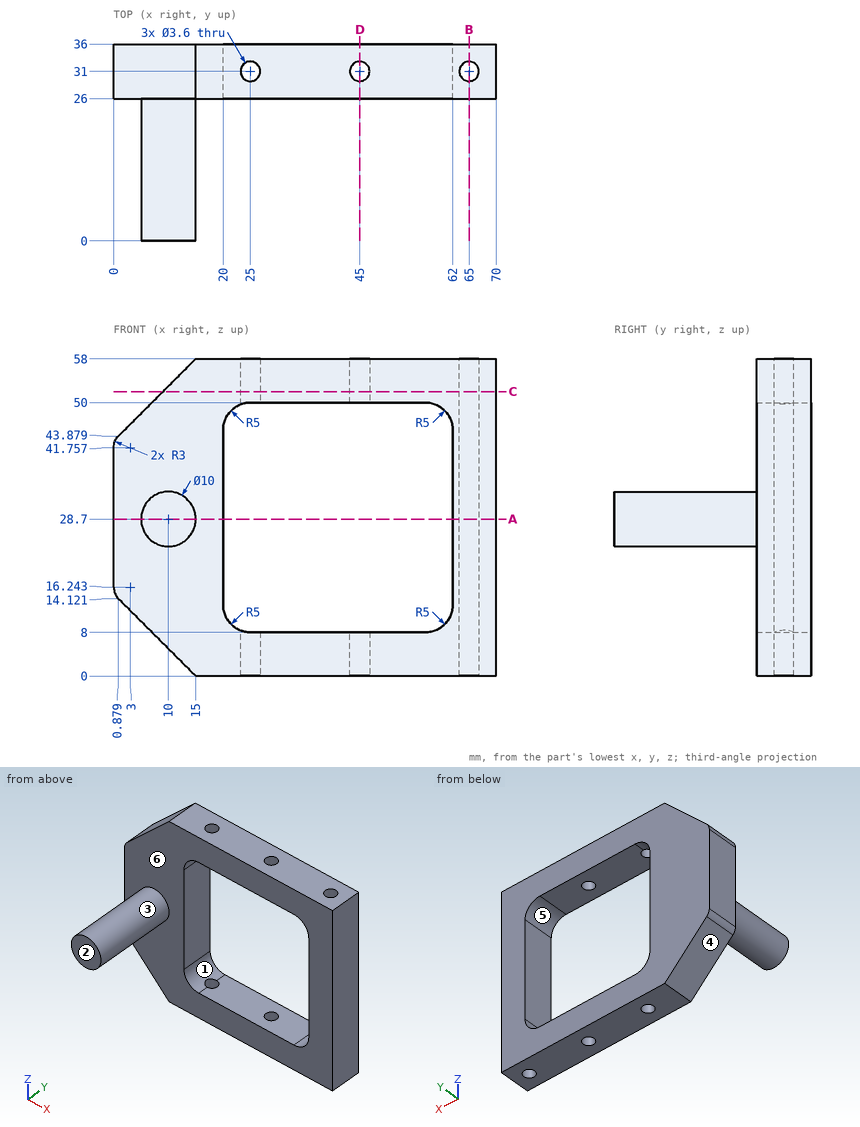
Verification items for this drawing (mm, ordinates from the low corner). A direction names the side the tool comes from. Round coordinates to 2 decimals unless told otherwise and drop trailing zeros. Loops run counter-clockwise (first coordinate to the right, second up) from the corner with the lowest first, then second, coordinate; pieces in that order, holes last. Notation, with made-up numbers: (22.25, 56.25) - (52.25, 56.25) arc R31 ccw to (52.25, 84.25) - close; hole circle Ø7 at (-28.5, 70). An arc over 180 degrees is marked (long way). Answer as CSV lines item,"result". Start each with the question number.
Item 1: Section check B-B (x = 65). Record the boundary of the cut face in (y, z), and give its area (3 significant figures).
Item 2: Section check A-A (z = 28.7). Record the boundary of the cut face in (x, y).
Item 3: Release check for a two-part mould opening along Z. For the marked faces 4, 5 and 6 record: +Z half, -Z half, draft (parallel to the pull), parting line (faces both ways), or undercut.
Item 4: Section check D-D (x = 45). Record the boundary of the cut face in (y, z).
Item 5: Scan lines: line 1 (Y direction, x = 45, z = 3.5); line 2 (X direction, y = 26.5, z = 34); line 3 (X direction, y = 31, z = 54). Record each from-to range of solid material in increasing order. Write a range as [from, to].
Item 6: Set-up check for the marked faces 1, 2 and 3: record each of +Z, -Z, +X, -X, +Y, -Y from which the full face is reachable in a straight line by a thin tool's end or side.
Item 7: Section check C-C (z = 52). Record the boundary of the cut face in (x, y).
Item 8: Depth check by flat-ended pin: P1, Ø3, axis at y = 23.5, z = 11, coming from the -X side; P2, Ø3, axis at x = 19.5, z = 39, coming from the -Y side; P3, Ø2, axis at y = 8, z = 29, coming from the -X side. Enter the tip coordinate at first touch or a pass-through.
Report:
1,outline,"(26, 0) - (29.2, 0) - (29.2, 58) - (26, 58) - close; (32.8, 0) - (36, 0) - (36, 58) - (32.8, 58) - close"
1,area,"371 mm2"
2,outline,"(0, 26) - (5, 26) - (5, 0) - (15, 0) - (15, 26) - (20, 26) - (20, 36) - (0, 36) - close; (62, 26) - (70, 26) - (70, 36) - (62, 36) - close; hole circle Ø3.6 at (65, 31)"
3,face 4,"-Z half"
3,face 5,"undercut"
3,face 6,"draft"
4,outline,"(26, 0) - (29.2, 0) - (29.2, 8) - (26, 8) - close; (26, 50) - (29.2, 50) - (29.2, 58) - (26, 58) - close; (32.8, 0) - (36, 0) - (36, 8) - (32.8, 8) - close; (32.8, 50) - (36, 50) - (36, 58) - (32.8, 58) - close"
5,line 1,"y = [26, 29.2], [32.8, 36]"
5,line 2,"x = [0, 20], [62, 70]"
5,line 3,"x = [11, 23.2], [26.8, 43.2], [46.8, 63.2], [66.8, 70]"
6,face 1,"+Y, -Y"
6,face 2,"+Z, -Z, +X, -X, -Y"
6,face 3,"-Y"
7,outline,"(9, 26) - (70, 26) - (70, 36) - (9, 36) - close; hole circle Ø3.6 at (25, 31); hole circle Ø3.6 at (45, 31); hole circle Ø3.6 at (65, 31)"
8,P1,"passes through"
8,P2,"stops at y = 26"
8,P3,"stops at x = 5"
